Read the model definition and answer for the solid it produces. Units are mm, in the model's axes. Round coordinates to 2 decimals unless told otherwise and drop trailing zeros. Write each loop counter-clockwise with the first axis right and the second up, starting at its lowest first coordinate (ties: lowest second). Pieces come first, ordered by that corner, then holes. Notation, with made-up numbers: (67.5, 55.5) - (74.5, 55.5) arc R19 cw to (74.5, 59.5) - close; hole circle Ø5 at (-6.5, 80.25). An arc over 180 degrees is marked (long way). One line per item, written item: value. Start each with the question number.
(1) The mould has two halves that part along X. Classify faces 1 (the face through (2349.221, 1804, -2)), 2 (the face through (2249.475, 1715.687, -1.972)), 3 (the face through (2285, 1914.5, -2)): +X half, -X half, draft (parallel to the pull), parting line (faces both ways), or undercut.
(2) A cutting plane is placed at B-B, the plane x = 2254. Determine the outline of the cut face in (y, z), plus the area to 3 significant figures.
(3) A cutting plane is placed at A-A, the plane x = 2318. Determine the outline of the cut face in (y, z).
(4) Find the intervals of material crossed by L1, parallel to X at y = 1892, z = -0.15; L2, parallel to Y at x = 2252.5, z = -0.25; L3, parallel to Y at x = 2257, z = -1.7, in increasing order.
from build123d import *

# Parameters (mm, degrees)
MODEL_W               = 126
MODEL_H               = 215
MODEL_R               = 4.5
MODEL_R_2             = 6.25
MODEL_R_3             = 2.25
TABAN_FLAN_1_DEPTH    = 4
IZIM1_W               = 106.122730642
IZIM1_H               = 29.615645761
SEKME1_DEPTH          = 4
IZIM4_R               = 4.25
KES_EKSTR_ZYON1_DEPTH = 10
RADYUS1_R             = 3


# Sheet-metal steps are written as plain solids
with BuildPart() as part:
    # Model → Taban-Flanş1 (new body)
    with BuildSketch(Plane.XY):
        with Locations((2286.221333619, 1807.000391939)):
            Rectangle(MODEL_W, MODEL_H)
        with Locations((2253.766329036, 1716.390896724)):
            Circle(MODEL_R, mode=Mode.SUBTRACT)
        with Locations((2318.766329036, 1716.390896724)):
            Circle(MODEL_R, mode=Mode.SUBTRACT)
        with Locations((2286.221329024, 1891.076796715)):
            Circle(MODEL_R_2, mode=Mode.SUBTRACT)
        with Locations((2236.221317757, 1891.076801538)):
            Circle(MODEL_R_3, mode=Mode.SUBTRACT)
        with Locations((2336.221317757, 1891.076801538)):
            Circle(MODEL_R_3, mode=Mode.SUBTRACT)
        with Locations((2237.221333619, 1850.077091939)):
            Circle(MODEL_R_3, mode=Mode.SUBTRACT)
        with Locations((2286.221333601, 1850.077091925)):
            Circle(MODEL_R_3, mode=Mode.SUBTRACT)
        with Locations((2335.22132399, 1850.077101041)):
            Circle(MODEL_R_3, mode=Mode.SUBTRACT)
    extrude(amount=-TABAN_FLAN_1_DEPTH)

    # Çizim1 → Sekme1 (add)
    with BuildSketch(Plane.XY):
        with Locations((2283.753363139, 1720.312928828)):
            Rectangle(IZIM1_W, IZIM1_H)
    extrude(amount=-SEKME1_DEPTH)

    # Çizim4 → Kes-Ekstrüzyon1 (cut)
    with BuildSketch(Plane.XY):
        with Locations((2253.721333619, 1715.500391939)):
            Circle(IZIM4_R)
        with Locations((2318.721333619, 1715.500391939)):
            Circle(IZIM4_R)
    extrude(amount=-KES_EKSTR_ZYON1_DEPTH, mode=Mode.SUBTRACT)

    # Radyus1
    radyus1_edges = [part.edges().sort_by_distance(p)[0] for p in [
        (2223.221333619, 1914.500391939, -2),
        (2349.221333619, 1914.500391939, -2),
    ]]
    fillet(radyus1_edges, radius=RADYUS1_R)


solid = part.part
Here are the results:
1. face 1: +X half
1. face 2: undercut
1. face 3: draft
2. outline: (1699.5, -4) - (1711.26, -4) - (1711.26, 0) - (1699.5, 0) - close; (1719.74, -4) - (1914.5, -4) - (1914.5, 0) - (1719.74, 0) - close
2. area: 826 mm²
3. outline: (1699.5, -4) - (1711.31, -4) - (1711.31, 0) - (1699.5, 0) - close; (1719.69, -4) - (1914.5, -4) - (1914.5, 0) - (1719.69, 0) - close
4. L1: 2223.22 to 2234.17, 2238.27 to 2280.04, 2292.4 to 2334.17, 2338.27 to 2349.22
4. L2: 1699.5 to 1711.43, 1719.57 to 1914.5
4. L3: 1699.5 to 1712.8, 1718.2 to 1914.5
